from build123d import *

# Parameters (mm, degrees)
SKETCH1_R           = 8.5
BOSS_EXTRUDE1_DEPTH = 7
BOSS_EXTRUDE2_DEPTH = 0.6
SKETCH3_R           = 5.8
CUT_EXTRUDE1_DEPTH  = 4.15


with BuildPart() as part:
    # Sketch1 → Boss-Extrude1 (new body)
    with BuildSketch(Plane.XY):
        Circle(SKETCH1_R)
    extrude(amount=BOSS_EXTRUDE1_DEPTH)

    # Sketch2 → Boss-Extrude2 (add)
    with BuildSketch(Plane.XY.offset(7)):
        with BuildLine():
            Line((-3.450980392, -1.394716626), (-0.617647059, 3.917783374))
            ThreePointArc((-0.617647059, 3.917783374), (0, 4.28837161), (0.617647059, 3.917783374))
            Line((0.617647059, 3.917783374), (3.450980392, -1.394716626))
            ThreePointArc((3.450980392, -1.394716626), (3.433578381, -2.084275419), (2.833333333, -2.42412839))
            Line((2.833333333, -2.42412839), (-2.833333333, -2.42412839))
            ThreePointArc((-2.833333333, -2.42412839), (-3.433578381, -2.084275419), (-3.450980392, -1.394716626))
        make_face()
    extrude(amount=BOSS_EXTRUDE2_DEPTH)

    # Sketch3 → Cut-Extrude1 (cut)
    with BuildSketch(Plane(origin=(0, 0, 0), x_dir=(-1, 0, 0), z_dir=(0, 0, -1))):
        Circle(SKETCH3_R)
    extrude(amount=-CUT_EXTRUDE1_DEPTH, mode=Mode.SUBTRACT)


solid = part.part
Verification items for the finished model (mm, model axes). A direction names the side the tool comes from. Give positions to 0.01 mm unless a question says otherwise; leave off trailing zeros. Loops run counter-clockwise (first coordinate to the right, second up) from the corner with the lowest first, then second, coordinate; pieces in that order, holes last.
1) Draft check along X on faces 4 (the cylindrical face through (5.794, 0.255, 2.046)), 5 (the flat face through (2.014, 1.299, 7.296)), 6 (the flat face through (0, 0, 7.6)). Enter one of: pulls with the +X half, pulls with the -X half, needs draft (parallel to the pull), parting line crosses it, or undercut.
2) Sectioned sample at A-A, the plane x = 0. Enter the section's corners in (y, z).
3) Sectioned sample at B-B, the plane y = -0.5. Enter the section's corners in (x, z), then the cut area to 3 significant figures.
4) Depth check by flat-ended pin: pin 1 Ø2 at (x, z) = (-1.5, 4.5) entering from -Y; pin 2 Ø1.5 at (y, z) = (-5.5, 1.5) entering from +X; pin 3 Ø9.5 at (x, y) = (0, 0) entering from -Z. Enter the tip coordinate at first touch or a pass-through.
5) Set-up check for faces 1 (the flat face through (2, 2, 7)), 2 (the flat face through (0, 0, 4.15)), 3 (the flat face through (-2.054, 1.224, 7.296)): record each of +Z, -Z, +X, -X, +Y, -Y from which the full face is reachable in a straight line by a thin tool's end or side.
6) Thickness scan on line 1 along Y through (x, z) = (0, 2.9); line 2 along Z through (x, y) = (0.5, 7.75); line 3 along Y through (x, z) = (-3.25, 2.75). Record the ranges inside material, lowest first.
7) Sectioned sample at D-D, the plane z = 4.75. Enter the section's corners in (x, y).
8) Sectioned sample at C-C, the plane z = 1. Enter the section's corners in (x, y).
Answers:
1. face 4: undercut
1. face 5: pulls with the +X half
1. face 6: needs draft
2. outline: (-8.5, 0) - (-5.8, 0) - (-5.8, 4.15) - (5.8, 4.15) - (5.8, 0) - (8.5, 0) - (8.5, 7) - (4.29, 7) - (4.29, 7.6) - (-2.42, 7.6) - (-2.42, 7) - (-8.5, 7) - close
3. outline: (-8.49, 0) - (-5.78, 0) - (-5.78, 4.15) - (5.78, 4.15) - (5.78, 0) - (8.49, 0) - (8.49, 7) - (2.97, 7) - (2.97, 7.6) - (-2.97, 7.6) - (-2.97, 7) - (-8.49, 7) - close
3. area: 74.4 mm2
4. pin 1: stops at y = -8.49
4. pin 2: stops at x = 7.05
4. pin 3: stops at z = 4.15
5. face 1: +Z
5. face 2: -Z
5. face 3: +Z, -X, +Y
6. line 1: y = -8.5 to -5.8, 5.8 to 8.5
6. line 2: z = 0 to 7
6. line 3: y = -7.85 to -4.8, 4.8 to 7.85
7. outline: circle Ø17 at (0, 0)
8. outline: circle Ø17 at (0, 0); hole circle Ø11.6 at (0, 0)
